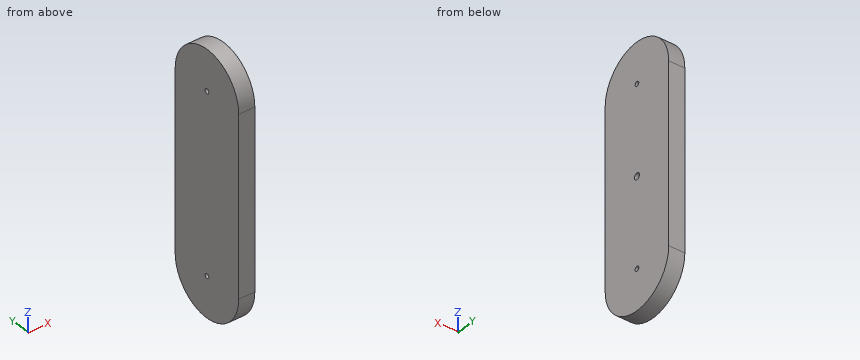
Autodesk Inventor part; units mm, degrees
ref_plane "YZ Plane" through (0, 0, 0) normal (1, 0, 0) x (0, 1, 0)
ref_plane "XZ Plane" through (0, 0, 0) normal (0, 1, 0) x (-1, 0, 0)
ref_plane "XY Plane" through (0, 0, 0) normal (0, 0, 1) x (1, 0, 0)
sketch "Sketch1" plane through (0, 0, 0) normal (1, 0, 0) x (0, 1, 0)
  arc A0 (4.9966, 65.5864) -> (36.7466, 65.5864) centre (20.8716, 65.5864) ccw
  line L0 (36.7466, 65.5864) -> (36.7466, 100.5114)
  line L1 (4.9966, 65.5864) -> (4.9966, 100.5114)
  arc A1 (36.7466, 135.4364) -> (4.9966, 135.4364) centre (20.8716, 135.4364) ccw
  line L2 (36.7466, 135.4364) -> (36.7466, 100.5114)
  line L3 (4.9966, 135.4364) -> (4.9966, 100.5114)
  circle A2 centre (20.8716, 135.4364) radius 0.9144
  circle A3 centre (20.8716, 65.5864) radius 0.9144
  dimension "d3" = 1.8288
  dimension "d4" = 1.8288
extrude "Extrusion1" add sketch "Sketch1" along normal blind 6.35
sketch "Sketch2" plane through (6.35, 0, 0) normal (1, 0, 0) x (0, 0, -1)
  point P0 (0, 0)
sketch "Sketch5" plane through (6.35, 0, 0) normal (1, 0, 0) x (0, 0, -1)
  circle A0 centre (-135.4364, 20.8716) radius 0.9144
  circle A1 centre (-65.5864, 20.8716) radius 0.9144
  circle A2 centre (-100.5114, 20.8716) radius 1.27
  point P0 (0, 0)
  dimension "d18" = 2.54
extrude "Extrusion4" cut sketch "Sketch5" against normal blind 2.9972 contours A2
properties part number "Second Arm half scale"
Source: CAD feature listing. Evaluate the final solid. Frame: model axes, mm. Give positions to 0.01 mm unless a question says otherwise; leave off trailing zeros. Loops run counter-clockwise (first coordinate to the right, second up) from the corner with the lowest first, then second, coordinate; pieces in that order, holes last. Notation, with made-up numbers: (-23.5, 75.5) -> (14.5, 75.5) arc R28 cw to (14.5, 108.5) -> close; hole circle Ø3 at (19, -29.75). An arc over 180 degrees is marked (long way). Use a Markdown table: item, result. Add a question column.
(1) Section query B-B (z = 56). Output: boundary loops of the cut face in (x, y), then the cut area to 3 significant figures.
(2) Section query C-C (y = 8.5). Output: boundary loops of the cut face in (x, z).
(3) First-contact query: pin 1 Ø3 at (x, y) = (5, 31) entering from -Z. Flat tip, straight axial feed; report the tip coordinate or a pass-through.
(4) Ray query, line 1 (Z direction, x = 0.75, y = 22); line 2 (Z direction, x = 5.75, y = 17); line 3 (Y direction, x = 5.5, z = 142). Return the intervals inside material, ascending.
(5) Section query A-A (x = 4.5). Output: boundary loops of the cut face in (y, z) (3 decimals).
Checked values:
| question | item | result |
|---|---|---|
| 1 | outline | (0, 8.22) -> (6.35, 8.22) -> (6.35, 33.53) -> (0, 33.53) -> close |
| 1 | area | 161 mm^2 |
| 2 | outline | (0, 55.64) -> (6.35, 55.64) -> (6.35, 145.38) -> (0, 145.38) -> close |
| 3 | pin 1 | z = 52.26 |
| 4 | line 1 | 49.75 to 151.27 |
| 4 | line 2 | 50.19 to 150.83 |
| 4 | line 3 | 6.42 to 35.33 |
| 5 | outline | (4.997, 65.586) arc R15.875 ccw to (36.747, 65.586) -> (36.747, 135.436) arc R15.875 ccw to (4.997, 135.436) -> close; hole circle Ø2.54 at (20.872, 100.511); hole circle Ø1.829 at (20.872, 65.586); hole circle Ø1.829 at (20.872, 135.436) |
